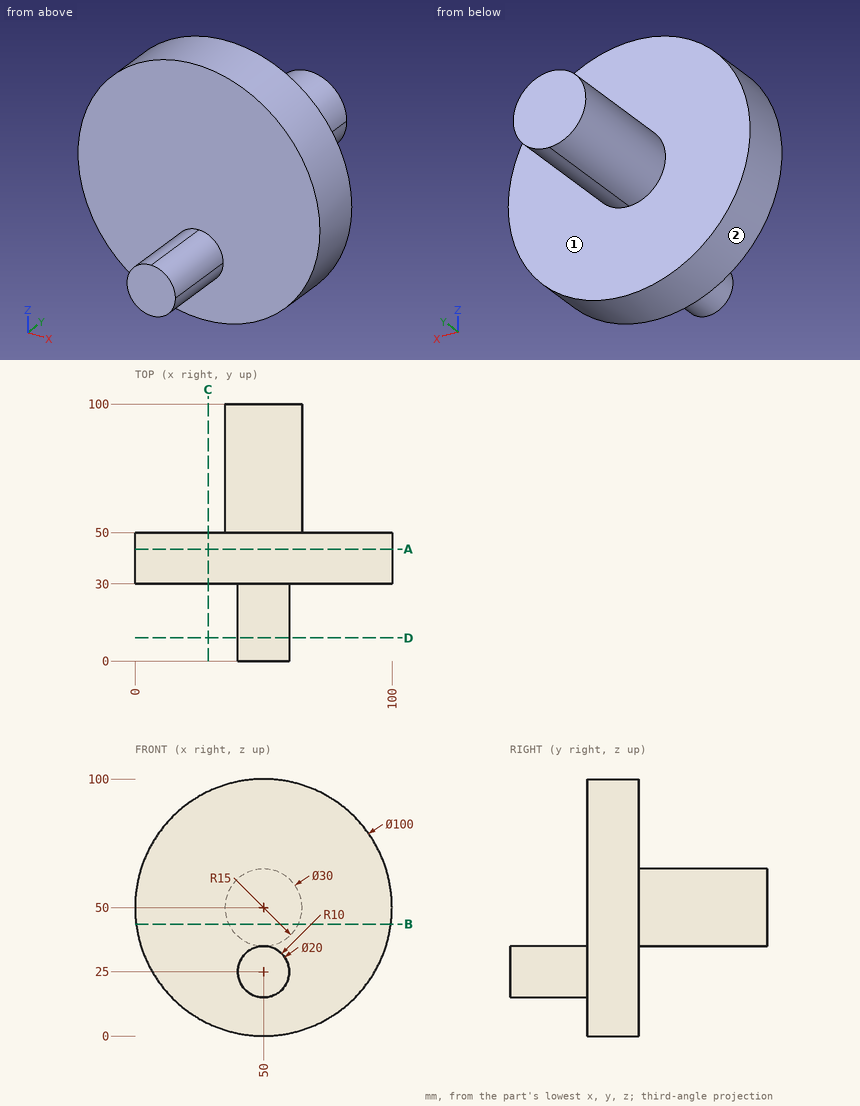
Geometry check sheet. Reference: drawing and pictorial views, mm from the part's lowest x, y, z. A direction names the side the tool comes from. Give positions to 0.01 mm unless a question says otherwise; leave off trailing zeros. Write each loop counter-clockwise with the first axis right and the second up, starting at its lowest first coordinate (ties: lowest second). Pieces come first, ordered by that corner, then holes. Notation, with made-up numbers: (7, 77.5) -> (40, 77.5) arc R21 ccw to (40, 101.5) -> close; hole circle Ø1 at (20.25, -29). An arc over 180 degrees is marked (long way). One line per item, written item: value. Start each with the question number.
Item 1: Section check A-A on y = 43.5. Record the cut outline in (x, z), then the cut area to 3 significant figures.
Item 2: Section check D-D on y = 9. Record the cut outline in (x, z).
Item 3: Gauge pin test, flat ends, axial feed: pin 1 (3 mm diameter, centred on x = 78, z = 88, fed in from +Y); pin 2 (8 mm diameter, centred on x = 67, z = 62.5, fed in from -Y); pin 3 (4 mm diameter, centred on y = 29, z = 76, fed in from +X); pin 4 (3 mm diameter, centred on y = 52.5, z = 77.5, fed in from +X). Record the tip position at first contact, or that the pin passes through.
Item 4: Section check C-C on x = 28.5. Record the cut outline in (y, z).
Item 5: Section check B-B on z = 43.5. Record the cut outline in (x, y), then the cut area to 3 significant figures.
Item 6: Tool access check on the marked faces 1 and 2. Record the directions out of +Z, -Z, +X, -X, +Y, -Y that give a thin tool (end or side, any length) a straight path to the whole face; none if there is none.
Item 7: Material ranges on probe 1 along Y at (x, z) = (48, 33.5); probe 2 along Y at (x, z) = (64, 43); probe 3 along X at (y, z) = (42, 49.5), recorded low to high. Write a range as from..to.
Results list:
1. outline: circle Ø100 at (50, 50)
1. area: 7,850 mm²
2. outline: circle Ø20 at (50, 25)
3. pin 1: y = 50
3. pin 2: y = 30
3. pin 3: x = 93.72
3. pin 4: through
4. outline: (30, 4.86) -> (50, 4.86) -> (50, 95.14) -> (30, 95.14) -> close
5. outline: (0.42, 30) -> (99.58, 30) -> (99.58, 50) -> (63.52, 50) -> (63.52, 100) -> (36.48, 100) -> (36.48, 50) -> (0.42, 50) -> close
5. area: 3,330 mm²
6. face 1: +Y
6. face 2: +Y, -Y
7. probe 1: 0..50
7. probe 2: 30..50
7. probe 3: 0..100
